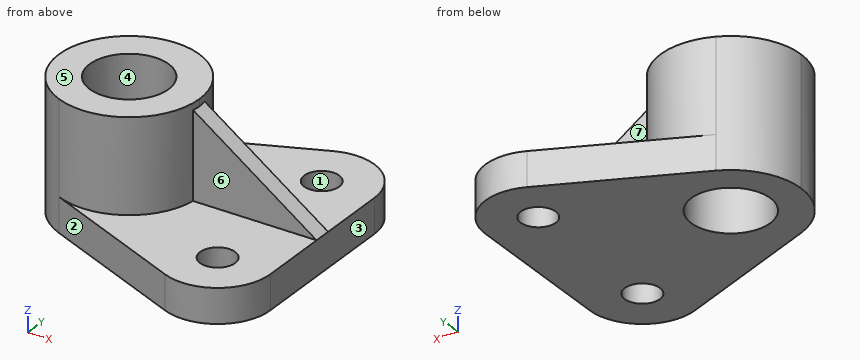
```python
from build123d import *

# Parameters (mm, degrees)
F0_R     = 14.2875
F1_DEPTH = 46.228
F0_R_2   = 6.35
F2_DEPTH = 12.446
F4_DEPTH = 3.175


with BuildPart() as f1:
    # F0 (on Top) → F1 (new body)
    with BuildSketch(Plane.XY):
        with BuildLine():
            ThreePointArc((-15.166243, 0), (-26.566113, 21.193309), (-50.532885, 23.36292))
            ThreePointArc((-50.532885, 23.36292), (-61.759552, 14.00013), (-65.966243, 0))
            ThreePointArc((-65.966243, 0), (-61.759552, -14.00013), (-50.532885, -23.36292))
            ThreePointArc((-50.532885, -23.36292), (-26.566113, -21.193309), (-15.166243, 0))
        make_face()
        with Locations((-40.566243, 0)):
            Circle(F0_R, mode=Mode.SUBTRACT)
    extrude(amount=F1_DEPTH)

    # F0 (on Top) → F2 (join)
    with BuildSketch(Plane.XY):
        with BuildLine():
            Line((29.283757, 0), (29.283757, 28.575))
            ThreePointArc((29.283757, 28.575), (20.733855, 44.469982), (2.758775, 46.09719))
            Line((2.758775, 46.09719), (-50.532885, 23.36292))
            ThreePointArc((-50.532885, 23.36292), (-26.566113, 21.193309), (-15.166243, 0))
            ThreePointArc((-15.166243, 0), (-26.566113, -21.193309), (-50.532885, -23.36292))
            Line((-50.532885, -23.36292), (2.758775, -46.09719))
            ThreePointArc((2.758775, -46.09719), (20.733855, -44.469982), (29.283757, -28.575))
            Line((29.283757, -28.575), (29.283757, 0))
        make_face()
        with Locations((10.233757, -28.575)):
            Circle(F0_R_2, mode=Mode.SUBTRACT)
        with Locations((10.233757, 28.575)):
            Circle(F0_R_2, mode=Mode.SUBTRACT)
    extrude(amount=F2_DEPTH)

    # F3 (on Front) → F4 (join, symmetric)
    with BuildSketch(Plane.XZ):
        Polygon((29.283757, 12.446), (-18.772896, 46.228), (-18.772896, 12.446), align=None)
    extrude(amount=F4_DEPTH, both=True)


solid = f1.part
```
The model under review builds one solid part; all positions refer to its coordinate system, in mm. Face numbers are marked on the shaded views. A direction names the side the tool comes from. Coordinates: 2 decimals unless noted, no trailing zeros. Order: outer loops, then holes, each group sorted by start corner. A loop starts at its lowest first (then second) coordinate and runs counter-clockwise, first axis right, second up. Notation, with made-up numbers: M -36,67.25 L -10,67.25 A16 ccw -10,78.25 Z; hole C 39.5,-6.75 d11. An arc over 180 degrees is marked long. One line per question, with ' | ' between items.
(1) Machinability: for the marked faces 5, 6 and 7, which of the approach directions +Z, -Z, +X, -X, +Y, -Y give a long, thin tool a straight path to every point of the face, cutting with its end or side? Answer none if there is none.
Geometry results:
face 5: +Z, +X, -X, +Y, -Y | face 6: +Z, +X, -Y | face 7: +Z, +X, +Y
(2) Add section C-C, the plane x = 6. Write out the cut boundary in (y, z) (3 decimals), then the cut area to 3 significant figures.
Geometry results:
outline: M -47.149,0 L -33.308,0 L -33.308,12.446 L -47.149,12.446 Z; M -23.842,0 L 23.842,0 L 23.842,12.446 L 3.175,12.446 L 3.175,28.814 L -3.175,28.814 L -3.175,12.446 L -23.842,12.446 Z; M 33.308,0 L 47.149,0 L 47.149,12.446 L 33.308,12.446 Z | area: 1,040 mm²
(3) Add section B-B, the plane y = -1.5. Write out the cut boundary in (x, z), then the cut area to 3 significant figures.
Geometry results:
outline: M -65.92,0 L -54.77,0 L -54.77,46.23 L -65.92,46.23 Z; M -26.36,0 L 29.28,0 L 29.28,12.45 L -15.21,43.72 L -15.21,46.23 L -26.36,46.23 Z | area: 2,280 mm²
(4) For probe 1 along Z at (x, y) = (-12.5, -21); probe 2 along X at (y, z) = (29.5, 7.5); probe 3 along X at (y, z) = (21, 35), list the stretches that pass through material, from the lowest coordinate up. Write a range as from..to.
Geometry results:
probe 1: z = 0..12.45 | probe 2: x = -36.15..3.95, 16.52..29.26 | probe 3: x = -54.85..-26.28
(5) Add section A-A, the plane z = 10.5. State how many separate pieces and enclosed holes the cut face has, then the cut area to 3 significant figures.
Geometry results:
separate pieces: 1 | enclosed holes: 3 | area: 5,690 mm²
(6) Insertion check: pin 1 (6 mm diameter, centred on y = -8, z = 31.5, fed in from +X); pin 2 (25 mm diameter, centred on x = -1, z = 30.5, fed in from +Y) (3 decimals); pin 3 (3 mm diameter, centred on x = -12, z = 41.5, fed in from -Y) (3 decimals). Each pin has a flat end and moves straight along its axis. Give the tip position at first contact, or say it passes through.
Geometry results:
pin 1: stops at x = -15.66 | pin 2: stops at y = 3.175 | pin 3: stops at y = -3.175
(7) The part is to be moulded in two halves that separate along X. For the marked faces 1, 2, 3 and 4, say which applies: +X half, -X half, draft (parallel to the pull), parting line (faces both ways), or undercut.
Geometry results:
face 1: undercut | face 2: -X half | face 3: +X half | face 4: undercut
(8) Add section D-D, the plane x = -29.5. Write out the cut boundary in (y, z).
Geometry results:
outline: M -32.34,0 L -9.04,0 L -9.04,46.23 L -22.86,46.23 L -22.86,12.45 L -32.34,12.45 Z; M 9.04,0 L 32.34,0 L 32.34,12.45 L 22.86,12.45 L 22.86,46.23 L 9.04,46.23 Z
